Could you check a few things on this drawing? It's one solid part, dimensions in mm from its lowest x, y, z. A direction names the side the tool comes from. Give positions to 0.01 mm unless a question says otherwise; leave off trailing zeros. Order: outer loops, then holes, each group sorted by start corner. A loop starts at its lowest first (then second) coordinate and runs counter-clockwise, first axis right, second up. Notation, with made-up numbers: (-37.75, 54) -> (-5.75, 54) arc R15 cw to (-5.75, 69) -> close; hole circle Ø1 at (77.25, 75). An arc over 180 degrees is marked (long way). Write each question's results on one line, items separated by ' | '.
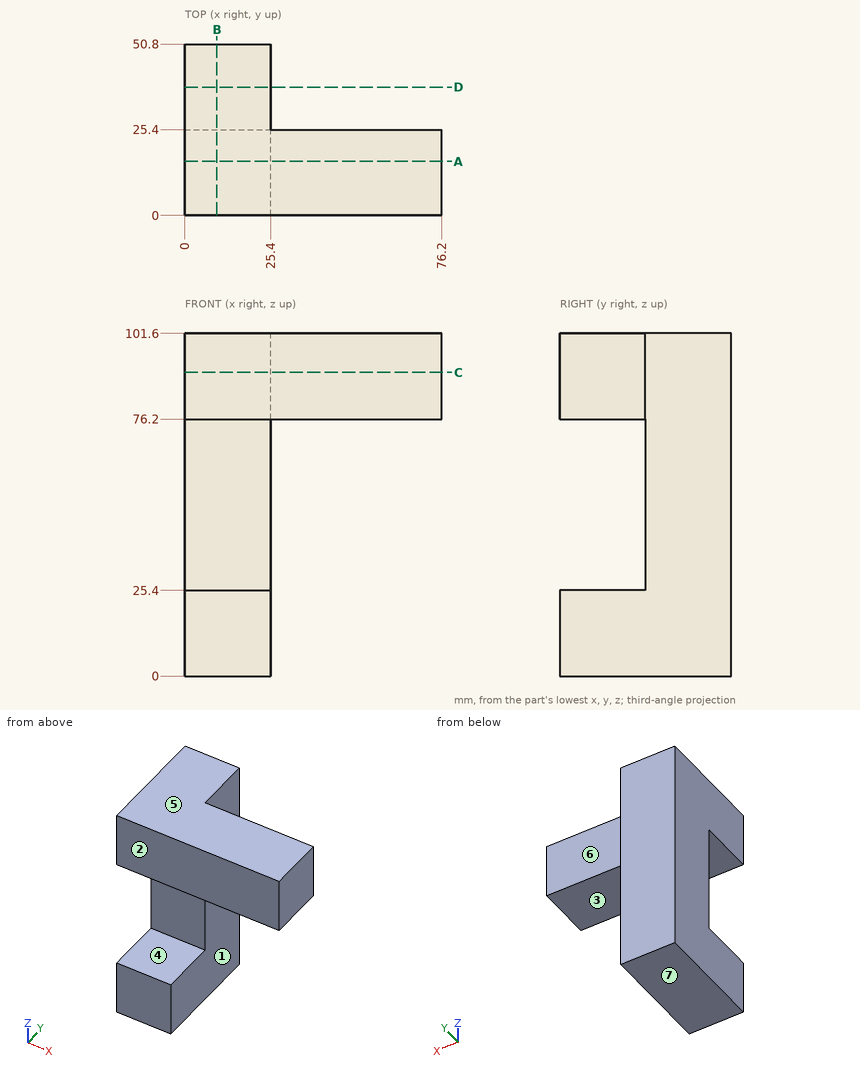
Q1. Suppose I cut it at C-C on z = 90. Please give me the cut outline in (x, y).
Here are the results:
outline: (0, 0) -> (76.2, 0) -> (76.2, 25.4) -> (25.4, 25.4) -> (25.4, 50.8) -> (0, 50.8) -> close
Q2. Suppose I cut it at B-B on x = 9.5. Please give me the cut outline in (y, z), and give its area (3 significant figures).
Here are the results:
outline: (0, 0) -> (50.8, 0) -> (50.8, 101.6) -> (0, 101.6) -> (0, 76.2) -> (25.4, 76.2) -> (25.4, 25.4) -> (0, 25.4) -> close | area: 3,870 mm²
Q3. Thinking about a two-plate mould opening in Z: for the marked faces 4, 5, 6 and 7, which applies, +Z half, -Z half, draft (parallel to the pull), parting line (faces both ways), or undercut?
Here are the results:
face 4: undercut | face 5: +Z half | face 6: draft | face 7: -Z half
Q4. Suppose I cut it at D-D on y = 38. Please give me the cut outline in (x, z), and give its area (3 significant figures).
Here are the results:
outline: (0, 0) -> (25.4, 0) -> (25.4, 101.6) -> (0, 101.6) -> close | area: 2,580 mm²
Q5. I need wall thicknesses on line 1 along X through (y, z) = (43.5, 22); line 2 along Z through (x, y) = (68, 15); line 3 along Y through (x, z) = (8, 72.5). Which ranges of each line are inside material? Lowest first, please.
Here are the results:
line 1: x = 0 to 25.4 | line 2: z = 76.2 to 101.6 | line 3: y = 25.4 to 50.8
Q6. For the marked faces 1, 2 and 3, which set-ups out of +Z, -Z, +X, -X, +Y, -Y let a thin tool reach every point of the face, with its end or its side?
Here are the results:
face 1: -Z, +X, +Y | face 2: +Z, -Z, +X, -X, -Y | face 3: +X, -X, -Y
Q7. Suppose I cut it at A-A on y = 16. Please give me the cut outline in (x, z), and give its area (3 significant figures).
Here are the results:
outline: (0, 0) -> (25.4, 0) -> (25.4, 25.4) -> (0, 25.4) -> close; (0, 76.2) -> (76.2, 76.2) -> (76.2, 101.6) -> (0, 101.6) -> close | area: 2,580 mm²
Q8. I'm going to push flat-ended pins straight in: pin 1 Ø1 at (x, y) = (32.5, 26.5) entering from +Z; pin 2 Ø2 at (y, z) = (39, 59.5) entering from +X; pin 3 Ø20.5 at (x, y) = (47, 15.5) entering from -Z; pin 4 Ø7.5 at (x, z) = (55, 94.5) entering from +Y. Where does each tip first touch, or does it pass through?
Here are the results:
pin 1: passes through | pin 2: stops at x = 25.4 | pin 3: stops at z = 76.2 | pin 4: stops at y = 25.4
